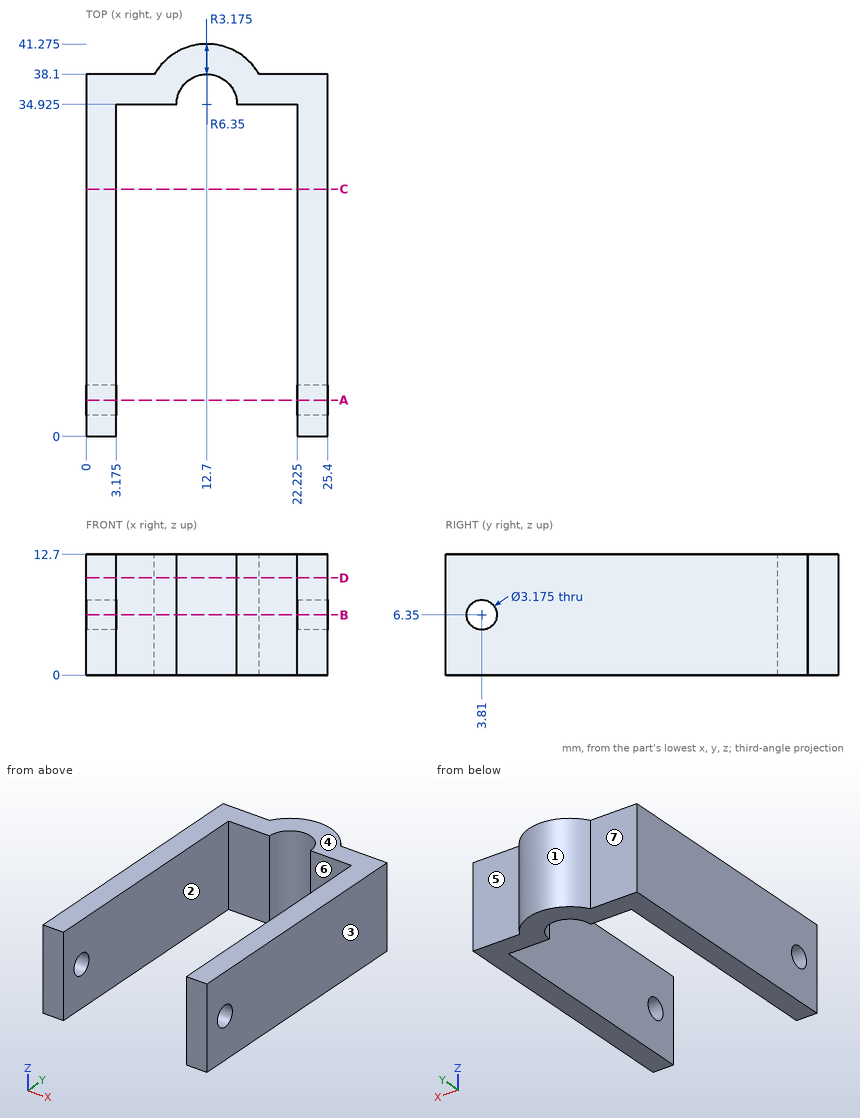
For this review, use the dimensioned drawing (mm, ordinates from the lowest corner) and the shaded views. A direction names the side the tool comes from. Round coordinates to 2 decimals unless told otherwise and drop trailing zeros. Write each loop counter-clockwise with the first axis right and the second up, starting at its lowest first coordinate (ties: lowest second). Pieces come first, ordered by that corner, then holes. Notation, with made-up numbers: (73.25, -37) - (85.25, -37) arc R25 ccw to (85.25, -1) - close; hole circle Ø6 at (-10.75, 68). An arc over 180 degrees is marked (long way). Answer as a JSON object with one key per item and string values.
1. Draft analysis for pull direction X (two halves, no side actions). For the marked faces 1, 2, 3 and 4, state which applies: +X half, -X half, draft (parallel to the pull), parting line (faces both ways), or undercut.
Response values:
{"face 1": "parting line", "face 2": "undercut", "face 3": "+X half", "face 4": "draft"}
2. We need section A-A on y = 3.81. Give the boundary of the cut face in (x, z) (1 decimal), then the cut area to 3 significant figures.
Response values:
{"outline": "(0, 0) - (3.2, 0) - (3.2, 4.8) - (0, 4.8) - close; (0, 7.9) - (3.2, 7.9) - (3.2, 12.7) - (0, 12.7) - close; (22.2, 0) - (25.4, 0) - (25.4, 4.8) - (22.2, 4.8) - close; (22.2, 7.9) - (25.4, 7.9) - (25.4, 12.7) - (22.2, 12.7) - close", "area": "60.5 mm2"}
3. Tool access review of the marked faces 5, 6 and 7: name each direction out of +Z, -Z, +X, -X, +Y, -Y from which nothing blocks a thin tool from reaching the whole face with its end or side.
Response values:
{"face 5": "+Z, -Z, +X, +Y", "face 6": "+Z, -Z, -Y", "face 7": "+Z, -Z, -X, +Y"}
4. For pin 1 Ø1.5 at (x, z) = (16, 4) entering from -Y (3 decimals); pin 2 Ø6 at (x, z) = (6.5, 3) entering from +Y; pin 3 Ø2 at (x, z) = (3, 5) entering from +Y; pin 4 Ø12 at (x, y) = (12.5, 21.5) entering from +Z, all flat-tipped, find the tip position at first contact; note any pin that passes through.
Response values:
{"pin 1": "stops at y = 34.925", "pin 2": "stops at y = 40.41", "pin 3": "stops at y = 38.1", "pin 4": "passes through"}
5. We need section D-D on z = 10.25. Give the boundary of the cut face in (x, y) (3 decimals), then the cut area to 3 significant figures.
Response values:
{"outline": "(0, 0) - (3.175, 0) - (3.175, 34.925) - (9.525, 34.925) arc R3.175 cw to (15.875, 34.925) - (22.225, 34.925) - (22.225, 0) - (25.4, 0) - (25.4, 38.1) - (18.199, 38.1) arc R6.35 ccw to (7.201, 38.1) - (0, 38.1) - close", "area": "311 mm2"}
6. We need section C-C on y = 26. Give the boundary of the cut face in (x, z) (3 decimals).
Response values:
{"outline": "(0, 0) - (3.175, 0) - (3.175, 12.7) - (0, 12.7) - close; (22.225, 0) - (25.4, 0) - (25.4, 12.7) - (22.225, 12.7) - close"}
7. We need section B-B on z = 6.35. Count the separate pieces of the cut face and the enclosed holes in it, then the cut area to 3 significant figures.
Response values:
{"separate pieces": "3", "enclosed holes": "0", "area": "291 mm2"}
8. To check wall thickness, follow line 1 along X through (y, z) = (3, 9) (3 decimals); line 2 along Y through (x, z) = (2.4, 6.35); line 3 along X through (y, z) = (35.5, 5.5). State the ranges of each line that lie inside material, in increasing order.
Response values:
{"line 1": "x = 0 to 3.175, 22.225 to 25.4", "line 2": "y = 0 to 2.22, 5.4 to 38.1", "line 3": "x = 0 to 9.58, 15.82 to 25.4"}
